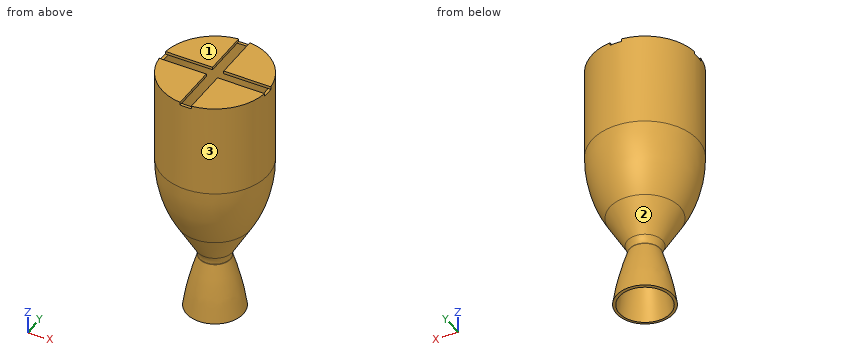
from build123d import *

# Parameters (mm, degrees)
SKETCH4_W          = 3.175
SKETCH4_H          = 12.7
CUT_EXTRUDE1_DEPTH = 298.085874974
CIRPATTERN1_COUNT  = 2
CIRPATTERN1_ANGLE  = 90


with BuildPart() as part:
    # Sketch2 → Revolve-Thin4 (revolve)
    with BuildSketch(Plane(origin=(0, 0, 0), x_dir=(0, 0, -1), z_dir=(1, 0, 0)), mode=Mode.PRIVATE) as revolve_thin4_sk:
        with BuildLine():
            Line((0, 0), (0, 56.769))
            Line((0, 56.769), (102.108, 56.769))
            ThreePointArc((102.108, 56.769), (140.500181874, 51.714573368), (176.276, 36.895744296))
            Line((176.276, 36.895744296), (210.593607924, 17.082464123))
            ThreePointArc((210.593607924, 17.082464123), (215.726112327, 14.954565751), (221.234, 14.224))
            ThreePointArc((221.234, 14.224), (222.082948, 14.290879198), (222.910433569, 14.49200893))
            ThreePointArc((222.910433569, 14.49200893), (253.5018987, 23.093142917), (284.734, 28.956))
            Line((284.734, 28.956), (284.286874616, 32.099358696))
            ThreePointArc((284.286874616, 32.099358696), (252.778619357, 26.184662284), (221.916664766, 17.507477147))
            ThreePointArc((221.916664766, 17.507477147), (221.581730132, 17.426067494), (221.238108322, 17.398997342))
            ThreePointArc((221.238108322, 17.398997342), (216.549846791, 18.020847951), (212.181107924, 19.83209478))
            Line((212.181107924, 19.83209478), (177.8635, 39.645374953))
            ThreePointArc((177.8635, 39.645374953), (141.321932343, 54.781387867), (102.108, 59.944))
            Line((102.108, 59.944), (-3.175, 59.944))
            Line((-3.175, 59.944), (-3.175, 0))
            Line((-3.175, 0), (0, 0))
        make_face()
    revolve(revolve_thin4_sk.sketch.rotate(Axis((0, 0, 0), (0, 0, -1)), 90), axis=Axis((0, 0, 0), (0, 0, -1)))

    # Sketch4 → Cut-Extrude1 (cut, symmetric)
    with BuildSketch(Plane(origin=(0, 0, 0), x_dir=(0, 0, -1), z_dir=(1, 0, 0))):
        with Locations((-1.5875, 0)):
            Rectangle(SKETCH4_W, SKETCH4_H)
    cut_extrude1 = extrude(amount=CUT_EXTRUDE1_DEPTH, both=True, mode=Mode.SUBTRACT)

    # CirPattern1: Cut-Extrude1 ×2 about axis
    cirpattern1_axis = Axis((0, 0, 3.175), (0, 0, 1))
    for i in range(1, CIRPATTERN1_COUNT):
        add(cut_extrude1.rotate(cirpattern1_axis, i * CIRPATTERN1_ANGLE / (CIRPATTERN1_COUNT - 1)), mode=Mode.SUBTRACT)


solid = part.part
The listing builds one solid part. Answer for the finished solid, in the listing's coordinates (mm). Face numbers are marked on the shaded views. Give positions to 0.01 mm unless a question says otherwise; leave off trailing zeros. Loops run counter-clockwise (first coordinate to the right, second up) from the corner with the lowest first, then second, coordinate; pieces in that order, holes last. Notation, with made-up numbers: M -27.75,-32 L 11.25,-32 A13 ccw 11.25,-25 Z; hole C -8.75,-28.75 d2. An arc over 180 degrees is marked long. Answer as CSV lines item,"result".
Item 1: The mould has two halves that part along Z. Classify the marked faces 1, 2 and 3: released by +Z, released by -Z, zero draft, split by the parting line, or undercut.
Values follow:
face 1,"released by +Z"
face 2,"undercut"
face 3,"zero draft"
Item 2: Straight lines are drawn through the part: line 1 along Y through (x, z) = (0, -63.5); line 2 along X through (y, z) = (17.5, -259); line 3 along Y through (x, z) = (25, -153). For each, find the intervals that lie inside material, in ascending order. Write a range as [from, to].
Values follow:
line 1,"y = [-59.94, -56.77], [56.77, 59.94]"
line 2,"x = [-21.32, -16.91], [16.91, 21.32]"
line 3,"y = [-44.61, -40.7], [40.7, 44.61]"
Item 3: The part is cut by section A-A (z = -191). Give the vertices of the cut face in (x, y).
Values follow:
outline,"C 0,0 d64.12; hole C 0,0 d56.79"
Item 4: Given pin 1 Ø10 at (x, y) = (44.5, 29.5) entering from -Z; pin 2 Ø1.8 at (x, y) = (-58, -3) entering from +Z; pin 3 Ø4 at (x, z) = (-17.5, -199.5) entering from -Y, each flat-ended and moving along its own axis, determine where each tip first touches the part or whether it passes through.
Values follow:
pin 1,"stops at z = -160.14"
pin 2,"stops at z = 0"
pin 3,"stops at y = -22.88"
